from build123d import *

# Parameters (mm, degrees)
SKETCH1_R              = 6
BOSS_EXTRUDE1_DEPTH    = 14
M5_TAPPED_HOLE1_REACH  = 48.435
M5_TAPPED_HOLE1_BORE_R = 2.1
CHAMFER1_SIZE          = 1


with BuildPart() as part:
    # Sketch1 → Boss-Extrude1 (new body)
    with BuildSketch(Plane.XY):
        with BuildLine():
            Line((-4.444097209, 19.5), (4.444097209, 19.5))
            ThreePointArc((4.444097209, 19.5), (14.142135624, -14.142135624), (-19.5, -4.444097209))
            Line((-19.5, -4.444097209), (-19.5, 4.444097209))
            ThreePointArc((-19.5, 4.444097209), (-14.142135624, 14.142135624), (-4.444097209, 19.5))
        make_face()
        Circle(SKETCH1_R, mode=Mode.SUBTRACT)
    extrude(amount=BOSS_EXTRUDE1_DEPTH)

    # M5 Tapped Hole1 bore → M5 Tapped Hole1 (cut, up to next)
    with BuildSketch(Plane(origin=(0, 19.5, 0), x_dir=(1, 0, 0), z_dir=(0, 1, 0)), mode=Mode.PRIVATE) as m5_tapped_hole1_sk1:
        with Locations((0, -7)):
            Circle(M5_TAPPED_HOLE1_BORE_R)
    m5_tapped_hole1_tool1 = extrude(m5_tapped_hole1_sk1.sketch, amount=-M5_TAPPED_HOLE1_REACH, mode=Mode.PRIVATE) & part.part
    add(m5_tapped_hole1_tool1.solids().sort_by_distance((0, 19.5, 7))[0], mode=Mode.SUBTRACT)

    # Chamfer1
    chamfer1_edges = [part.edges().sort_by_distance(p)[0] for p in [
        (14.142135624, -14.142135624, 0),
    ]]
    chamfer(chamfer1_edges, length=CHAMFER1_SIZE)
    chamfer1_2_edges = [part.edges().sort_by_distance(p)[0] for p in [
        (14.142135624, -14.142135624, 14),
    ]]
    chamfer(chamfer1_2_edges, length=CHAMFER1_SIZE)
    chamfer1_3_edges = [part.edges().sort_by_distance(p)[0] for p in [
        (-14.142135624, 14.142135624, 0),
    ]]
    chamfer(chamfer1_3_edges, length=CHAMFER1_SIZE - 0.0001)  # a hair under: the kernel refuses the full size
    chamfer1_4_edges = [part.edges().sort_by_distance(p)[0] for p in [
        (-14.142135624, 14.142135624, 14),
    ]]
    chamfer(chamfer1_4_edges, length=CHAMFER1_SIZE - 0.0001)  # a hair under: the kernel refuses the full size


solid = part.part
Design review of the part built by this model. Coordinates are the model's own, in mm. A direction names the side the tool comes from. Coordinates: 2 decimals unless noted, no trailing zeros. Write each loop counter-clockwise with the first axis right and the second up, starting at its lowest first coordinate (ties: lowest second). Pieces come first, ordered by that corner, then holes. Notation, with made-up numbers: (10.5, 31) - (19.5, 31) arc R15 ccw to (19.5, 54) - close; hole circle Ø11 at (-24, 33.5). An arc over 180 degrees is marked (long way). Use one line per item in the form item = value.
Q1. Machinability: for faces 4 (the conical face through (13.956, -13.147, 0.174)), 5 (the cylindrical face through (-0.273, 12.657, 4.918)), which of the approach directions +Z, -Z, +X, -X, +Y, -Y give a long, thin tool a straight path to every point of the face, cutting with its end or side? Answer none if there is none.
Taken from the geometry:
face_4 = -Z
face_5 = +Y
Q2. Insertion check: pin 1 Ø1.5 at (y, z) = (6.5, 8) entering from -X; pin 2 Ø8 at (x, z) = (-13, 12.5) entering from +Y; pin 3 Ø8 at (y, z) = (7.5, 3.5) entering from +X. Each pin has a flat end and moves straight along its axis. Give the tip position at first contact, or say it passes through.
Taken from the geometry:
pin_1 = -19.16
pin_2 = 17.86
pin_3 = 19.69
Q3. Consider section B-B (y = 0). Write out the cut boundary in (x, z).
Taken from the geometry:
outline = (-19.5, 0.5) - (-19, 0) - (-6, 0) - (-6, 14) - (-19, 14) - (-19.5, 13.5) - close; (6, 0) - (19, 0) - (20, 1) - (20, 13) - (19, 14) - (6, 14) - close
Q4. Consider section D-D (z = 11.5). Write out the cut boundary in (x, y), plus the area to 3 significant figures.
Taken from the geometry:
outline = (-19.5, -4.44) arc R20 ccw (long way) to (4.44, 19.5) - (-4.44, 19.5) arc R20 ccw to (-19.5, 4.44) - close; hole circle Ø12 at (0, 0)
area = 1,140 mm^2
Q5. Consider section A-A (x = 0). Write out the cut boundary in (y, z), plus the area to 3 significant figures.
Taken from the geometry:
outline = (-20, 1) - (-19, 0) - (-6, 0) - (-6, 14) - (-19, 14) - (-20, 13) - close; (6, 0) - (19, 0) - (19.5, 0.5) - (19.5, 4.9) - (6, 4.9) - close; (6, 9.1) - (19.5, 9.1) - (19.5, 13.5) - (19, 14) - (6, 14) - close
area = 327 mm^2
Q6. The part is to be moulded in two halves that separate along X. For faces 1 (the flat face through (-2, 19.5, 5)), 2 (the conical face through (13.946, -13.138, 13.84)), 3 (the cylindrical face through (-1.301, -5.857, 6.902)), say which applies: +X half, -X half, draft (parallel to the pull), parting line (faces both ways), or undercut.
Taken from the geometry:
face_1 = draft
face_2 = parting line
face_3 = undercut
Q7. For probe 1 along Y at (x, z) = (0, 9.25); probe 2 along Z at (x, y) = (0, 14); probe 3 along X at (y, z) = (9.5, 7), list the stretches that pass through material, from the lowest coordinate up.
Taken from the geometry:
probe_1 = -20 to -6, 6 to 19.5
probe_2 = 0 to 4.9, 9.1 to 14
probe_3 = -17.6 to -2.1, 2.1 to 17.6
Q8. Consider section C-C (z = 7). Write out the cut boundary in (x, y).
Taken from the geometry:
outline = (-19.5, -4.44) arc R20 ccw (long way) to (4.44, 19.5) - (2.1, 19.5) - (2.1, 5.62) arc R6 cw (long way) to (-2.1, 5.62) - (-2.1, 19.5) - (-4.44, 19.5) arc R20 ccw to (-19.5, 4.44) - close
